Could you check a few things on this model? Use its own coordinates, in mm. A direction names the side the tool comes from. Round coordinates to 2 decimals unless told otherwise and drop trailing zeros. Loops run counter-clockwise (first coordinate to the right, second up) from the corner with the lowest first, then second, coordinate; pieces in that order, holes last. Notation, with made-up numbers: (29, 44) -> (73, 44) arc R28 ccw to (73, 67) -> close; hole circle Ø3 at (23, 75.5). An arc over 180 degrees is marked (long way). One line per item, written item: value.
```python
from build123d import *

# Parameters (mm, degrees)
SKETCH_1_W          = 3
SKETCH_1_H          = 7
SKETCH_1_W_2        = 12
SKETCH_1_H_2        = 12
SKETCH_1_W_3        = 7
SKETCH_1_W_4        = 5
EXTRUDE_1_DEPTH     = 9
CUT_EXTRUDE_1_DEPTH = 17.911534525
FILLET_1_R          = 4.5
SKETCH_3_R          = 1.5
CUT_EXTRUDE_2_DEPTH = 19.445866746
FILLET_2_R          = 3
SKETCH_4_R          = 1.5
CUT_EXTRUDE_3_DEPTH = 19.193405399
FILLET_3_R          = 1
FILLET_4_R          = 1
FILLET_5_R          = 1
FILLET_6_R          = 1


# Some blends are built 0.0001 mm under size
with BuildPart() as part:
    # 草图1 → 凸台-拉伸1 (new body)
    # profile 1 of 4: a face of its own
    with BuildSketch(Plane.XY):
        with Locations((-1.5, 9.5)):
            Rectangle(SKETCH_1_W, SKETCH_1_H)
    # profile 2 of 4: a face of its own
    with BuildSketch(Plane.XY):
        with Locations((1.5, 9.5)):
            Rectangle(SKETCH_1_W, SKETCH_1_H)
    # profile 3 of 4: a face of its own
    with BuildSketch(Plane.XY):
        Rectangle(SKETCH_1_W_2, SKETCH_1_H_2)
        Rectangle(SKETCH_1_W_3, SKETCH_1_H, mode=Mode.SUBTRACT)
    # profile 4 of 4: a face of its own
    with BuildSketch(Plane.XY):
        with Locations((1, -9.5)):
            Rectangle(SKETCH_1_W_4, SKETCH_1_H)
    extrude(amount=EXTRUDE_1_DEPTH)

    # 草图2 → 切除-拉伸1 (cut, through all)
    with BuildSketch(Plane.XY.offset(9)):
        Polygon((0, 13), (0.4, 13), (0.4, 3.5), (0, 3.5), (-0.4, 3.5), (-0.4, 13), align=None)
    extrude(amount=-CUT_EXTRUDE_1_DEPTH, mode=Mode.SUBTRACT)

    # 圆角1
    fillet_1_edges = [part.edges().sort_by_distance(p)[0] for p in [
        (1, -13, 0),
        (1, -13, 9),
    ]]
    fillet(fillet_1_edges, radius=FILLET_1_R - 0.0001)  # a hair under: the kernel refuses the full size

    # 草图3 → 切除-拉伸2 (cut, through all)
    with BuildSketch(Plane(origin=(3.5, 0, 0), x_dir=(0, 0, -1), z_dir=(1, 0, 0))):
        with Locations(Location((-4.5, -9.5, 0), (0, 0, 90))):
            Circle(SKETCH_3_R)
    extrude(amount=-CUT_EXTRUDE_2_DEPTH, mode=Mode.SUBTRACT)

    # 圆角2
    fillet_2_edges = [part.edges().sort_by_distance(p)[0] for p in [
        (1.7, 13, 9),
        (1.7, 13, 0),
        (-1.7, 13, 0),
        (-1.7, 13, 9),
    ]]
    fillet(fillet_2_edges, radius=FILLET_2_R)

    # 草图4 → 切除-拉伸3 (cut, through all)
    with BuildSketch(Plane(origin=(3, 0, 0), x_dir=(0, 0, -1), z_dir=(1, 0, 0))):
        with Locations((-4.5, 9.5)):
            Circle(SKETCH_4_R)
    extrude(amount=-CUT_EXTRUDE_3_DEPTH, mode=Mode.SUBTRACT)

    # 圆角3
    fillet_3_edges = [part.edges().sort_by_distance(p)[0] for p in [
        (3, 12.121320344, 8.121320344),
        (3, 12.121320344, 0.878679656),
        (3, 8, 9),
        (6, 0, 0),
        (3, 8, 0),
        (4.5, 6, 0),
        (6, 6, 4.5),
        (6, -6, 4.5),
        (4.5, 6, 9),
        (6, 0, 9),
        (3, 13, 4.5),
    ]]
    fillet(fillet_3_edges, radius=FILLET_3_R)

    # 圆角4
    fillet_4_edges = [part.edges().sort_by_distance(p)[0] for p in [
        (-3, 13, 4.5),
        (-3, 12.121320344, 8.121320344),
        (-3, 12.121320344, 0.878679656),
        (-3, 8, 9),
        (-6, 0, 0),
        (-4.5, 6, 0),
        (-3, 8, 0),
        (-4.5, 6, 9),
        (-6, 0, 9),
        (-6, -6, 4.5),
    ]]
    fillet(fillet_4_edges, radius=FILLET_4_R)

    # 圆角5
    # the kernel refuses this fillet: 1 mm, written as the material it takes off along each edge
    with BuildSketch(Plane(origin=(-5, 5, 8), x_dir=(0, 1, 0), z_dir=(-1, 0, 0))) as fillet_5_piece_1_section:
        Polygon((0, 0), (FILLET_5_R, 0), (FILLET_5_R, -FILLET_5_R), (0, -FILLET_5_R), align=None)
    fillet_5_piece_1 = extrude(amount=FILLET_5_R, mode=Mode.PRIVATE)
    fillet_5_piece_1 = fillet_5_piece_1 - Plane(origin=(-5, 5, 8), x_dir=(0, -0.7071067811865475, -0.7071067811865475), z_dir=(-1, 0, 0)) * Sphere(FILLET_5_R, mode=Mode.PRIVATE)
    add(fillet_5_piece_1, mode=Mode.SUBTRACT)
    with BuildSketch(Plane(origin=(-5, 5, 1), x_dir=(0, 1, 0), z_dir=(-1, 0, 0))) as fillet_5_piece_2_section:
        Polygon((0, 0), (FILLET_5_R, 0), (FILLET_5_R, FILLET_5_R), (0, FILLET_5_R), align=None)
    fillet_5_piece_2 = extrude(amount=FILLET_5_R, mode=Mode.PRIVATE)
    fillet_5_piece_2 = fillet_5_piece_2 - Plane(origin=(-5, 5, 1), x_dir=(0, -0.7071067811865475, 0.7071067811865475), z_dir=(-1, 0, 0)) * Sphere(FILLET_5_R, mode=Mode.PRIVATE)
    add(fillet_5_piece_2, mode=Mode.SUBTRACT)
    with BuildSketch(Plane(origin=(-6, 6, 1), x_dir=(0, -1, 0), z_dir=(0, 0, 1))) as fillet_5_piece_3:
        with BuildLine():
            CenterArc((FILLET_5_R, FILLET_5_R), FILLET_5_R, 180, 90)
            Line((0, FILLET_5_R), (0, 0))
            Line((0, 0), (FILLET_5_R, 0))
        make_face()
    extrude(amount=7, mode=Mode.SUBTRACT)

    # 圆角6
    # the kernel refuses this fillet: 1 mm, written as the material it takes off along each edge
    with BuildSketch(Plane(origin=(5, -5, 8), x_dir=(0, 0, 1), z_dir=(0, -1, 0))) as fillet_6_piece_1_section:
        Polygon((0, 0), (FILLET_6_R, 0), (FILLET_6_R, -FILLET_6_R), (0, -FILLET_6_R), align=None)
    fillet_6_piece_1 = extrude(amount=FILLET_6_R, mode=Mode.PRIVATE)
    fillet_6_piece_1 = fillet_6_piece_1 - Plane(origin=(5, -5, 8), x_dir=(-0.7071067811865475, 0, -0.7071067811865475), z_dir=(0, -1, 0)) * Sphere(FILLET_6_R, mode=Mode.PRIVATE)
    add(fillet_6_piece_1, mode=Mode.SUBTRACT)
    with BuildSketch(Plane(origin=(5, -5, 1), x_dir=(0, -1, 0), z_dir=(0, 0, -1))) as fillet_6_piece_2_section:
        Polygon((0, 0), (FILLET_6_R, 0), (FILLET_6_R, -FILLET_6_R), (0, -FILLET_6_R), align=None)
    fillet_6_piece_2 = extrude(amount=FILLET_6_R, mode=Mode.PRIVATE)
    fillet_6_piece_2 = fillet_6_piece_2 - Plane(origin=(5, -5, 1), x_dir=(-0.7071067811865476, 0.7071067811865475, 0), z_dir=(0, 0, -1)) * Sphere(FILLET_6_R, mode=Mode.PRIVATE)
    add(fillet_6_piece_2, mode=Mode.SUBTRACT)
    with BuildSketch(Plane(origin=(5, -6, 0), x_dir=(0, 1, 0), z_dir=(-1, 0, 0)), Plane(origin=(5, -6, 9), x_dir=(0, 0, -1), z_dir=(-1, 0, 0))) as fillet_6_piece_3:
        with BuildLine():
            CenterArc((FILLET_6_R, -FILLET_6_R), FILLET_6_R, 90, 90)
            Line((0, -FILLET_6_R), (0, 0))
            Line((0, 0), (FILLET_6_R, 0))
        make_face()
    extrude(amount=1.5, mode=Mode.SUBTRACT)
    with BuildSketch(Plane(origin=(3.5, -8.5001, 0), x_dir=(-1, 0, 0), z_dir=(0, 1, 0)), Plane(origin=(3.5, -8.5001, 9), x_dir=(0, 0, -1), z_dir=(0, 1, 0))) as fillet_6_piece_4:
        with BuildLine():
            CenterArc((FILLET_6_R, FILLET_6_R), FILLET_6_R, 180, 90)
            Line((0, FILLET_6_R), (0, 0))
            Line((0, 0), (FILLET_6_R, 0))
        make_face()
    extrude(amount=2.5001, mode=Mode.SUBTRACT)
    with BuildSketch(Plane(origin=(3.5, -8.5001, 4.5001), x_dir=(0, 0, 1), z_dir=(0, 1, 0))) as fillet_6_piece_5:
        with BuildLine():
            CenterArc((4.4999 - FILLET_6_R, -FILLET_6_R), FILLET_6_R, 0, 90)
            Line((4.4999, -FILLET_6_R), (4.4999, 0))
            Line((4.4999, 0), (4.4999 - FILLET_6_R, 0))
        make_face()
    revolve(axis=Axis((3.5, -8.5001, 4.5001), (1, 0, 0)), revolution_arc=90, mode=Mode.SUBTRACT)
    with BuildSketch(Plane(origin=(3.5, -8.5001, 4.4999), x_dir=(0, 0, -1), z_dir=(0, 1, 0))) as fillet_6_piece_6:
        with BuildLine():
            CenterArc((4.4999 - FILLET_6_R, FILLET_6_R), FILLET_6_R, 270, 90)
            Line((4.4999 - FILLET_6_R, 0), (4.4999, 0))
            Line((4.4999, 0), (4.4999, FILLET_6_R))
        make_face()
    revolve(axis=Axis((3.5, -8.5001, 4.4999), (-1, 0, 0)), revolution_arc=90, mode=Mode.SUBTRACT)
    with BuildSketch(Plane(origin=(3.5, -13, 4.4999), x_dir=(0, 1, 0), z_dir=(0, 0, 1))) as fillet_6_piece_7:
        with BuildLine():
            CenterArc((FILLET_6_R, FILLET_6_R), FILLET_6_R, 180, 90)
            Line((0, FILLET_6_R), (0, 0))
            Line((0, 0), (FILLET_6_R, 0))
        make_face()
    extrude(amount=0.0002, mode=Mode.SUBTRACT)
    with BuildSketch(Plane(origin=(3.5, -8.5001, 0), x_dir=(-1, 0, 0), z_dir=(0, 1, 0))) as fillet_6_piece_8a_section:
        with BuildLine():
            CenterArc((FILLET_6_R, FILLET_6_R), FILLET_6_R, 180, 90)
            Line((0, FILLET_6_R), (0, 0))
            Line((0, 0), (FILLET_6_R, 0))
        make_face()
    fillet_6_piece_8a = extrude(amount=5.0001, mode=Mode.PRIVATE)
    fillet_6_piece_8a = split(fillet_6_piece_8a, bisect_by=Plane(origin=(3.273604886, -6, 0.226395114), z_dir=(0, 1, 0)), keep=Keep.TOP, mode=Mode.PRIVATE)
    with BuildSketch(Plane(origin=(5, -6, 0), x_dir=(0, 1, 0), z_dir=(-1, 0, 0))) as fillet_6_piece_8b_section:
        with BuildLine():
            CenterArc((FILLET_6_R, -FILLET_6_R), FILLET_6_R, 90, 90)
            Line((0, -FILLET_6_R), (0, 0))
            Line((0, 0), (FILLET_6_R, 0))
        make_face()
    fillet_6_piece_8b = extrude(amount=4, mode=Mode.PRIVATE)
    fillet_6_piece_8b = split(fillet_6_piece_8b, bisect_by=Plane(origin=(3.5, -5.773604886, 0.226395114), z_dir=(-1, 0, 0)), keep=Keep.TOP, mode=Mode.PRIVATE)
    fillet_6_piece_8 = fillet_6_piece_8a & fillet_6_piece_8b
    add(fillet_6_piece_8, mode=Mode.SUBTRACT)
    with BuildSketch(Plane(origin=(3.5, -8.5001, 9), x_dir=(0, 0, -1), z_dir=(0, 1, 0))) as fillet_6_piece_9a_section:
        with BuildLine():
            CenterArc((FILLET_6_R, FILLET_6_R), FILLET_6_R, 180, 90)
            Line((0, FILLET_6_R), (0, 0))
            Line((0, 0), (FILLET_6_R, 0))
        make_face()
    fillet_6_piece_9a = extrude(amount=5.0001, mode=Mode.PRIVATE)
    fillet_6_piece_9a = split(fillet_6_piece_9a, bisect_by=Plane(origin=(3.273604886, -6, 8.773604886), z_dir=(0, 1, 0)), keep=Keep.TOP, mode=Mode.PRIVATE)
    with BuildSketch(Plane(origin=(5, -6, 9), x_dir=(0, 0, -1), z_dir=(-1, 0, 0))) as fillet_6_piece_9b_section:
        with BuildLine():
            CenterArc((FILLET_6_R, -FILLET_6_R), FILLET_6_R, 90, 90)
            Line((0, -FILLET_6_R), (0, 0))
            Line((0, 0), (FILLET_6_R, 0))
        make_face()
    fillet_6_piece_9b = extrude(amount=4, mode=Mode.PRIVATE)
    fillet_6_piece_9b = split(fillet_6_piece_9b, bisect_by=Plane(origin=(3.5, -5.773604886, 8.773604886), z_dir=(-1, 0, 0)), keep=Keep.TOP, mode=Mode.PRIVATE)
    fillet_6_piece_9 = fillet_6_piece_9a & fillet_6_piece_9b
    add(fillet_6_piece_9, mode=Mode.SUBTRACT)


solid = part.part
```
(1) For pin 1 Ø0.6 at (x, z) = (-4, 3.5) entering from +Y; pin 2 Ø3.5 at (y, z) = (-9.5, 4.5) entering from -X; pin 3 Ø2 at (x, z) = (3.5, 6) entering from +Y, each with a flat end and sliding along its axis, tell me the tip position at first contact or that it passes through.
Results below:
pin 1: stops at y = 6
pin 2: stops at x = -1.5
pin 3: stops at y = 12.87
(2) Imagine slicing it at B-B on y = 9.5. Write out the boundary of the cut face in (x, z), then the cut area to 3 significant figures.
Results below:
outline: (-3, 1) arc R1 ccw to (-2, 0) -> (-0.4, 0) -> (-0.4, 3) -> (-3, 3) -> close; (-3, 6) -> (-0.4, 6) -> (-0.4, 9) -> (-2, 9) arc R1 ccw to (-3, 8) -> close; (0.4, 0) -> (2, 0) arc R1 ccw to (3, 1) -> (3, 3) -> (0.4, 3) -> close; (0.4, 6) -> (3, 6) -> (3, 8) arc R1 ccw to (2, 9) -> (0.4, 9) -> close
area: 30.3 mm²
(3) On a 3-axis mill with a long thin cutter (end or side, diameter ignored), from which of +Z, -Z, +X, -X, +Y, -Y can I reach the whole of each face in a straight line? I mean faces 1 (the face through (0, -3.5, 4)), 2 (the face through (-2.715, 8.091, 0.301)), 3 (the face through (-3, -6, 4)), 4 (the face through (2.715, 8.091, 0.301)). Say none if no direction works.
Results below:
face 1: +Z, -Z
face 2: -Z, -X, +Y
face 3: +Z, -Z, -X, -Y
face 4: -Z, +X, +Y
(4) Imagine slicing it at A-A on x = 0.75. Give the number of separate pieces and of enclosed holes in the cut face, then the cut area to 3 significant figures.
Results below:
separate pieces: 2
enclosed holes: 2
area: 144 mm²
(5) Please list where these lines run through material, in increasing order: L1, parallel to X at y = 9, z = 6; L2, parallel to Y at x = -1.75, z = 4.25; L3, parallel to X at y = -3, z = 6.
Results below:
L1: x = -3 to -0.4, 0.4 to 3
L2: y = -6 to -3.5, 3.5 to 8.02, 10.98 to 13
L3: x = -6 to -3.5, 3.5 to 6
(6) Imagine slicing it at D-D on y = -5.5. Write out the boundary of the cut face in (x, z).
Results below:
outline: (-5.87, 0.5) arc R1 ccw to (-5, 0) -> (2.5, 0) arc R1 ccw to (3, 0.13) -> (5, 0.13) arc R0.87 ccw to (5.87, 1) -> (5.87, 8) arc R0.87 ccw to (5, 8.87) -> (3, 8.87) arc R1 ccw to (2.5, 9) -> (-5, 9) arc R1 ccw to (-5.87, 8.5) -> close
